Check sheet for the modelled part. Datum: model origin and axes. Units: mm. A direction names the side the tool comes from. Round coordinates to 2 decimals unless told otherwise and drop trailing zeros. Order: outer loops, then holes, each group sorted by start corner. A loop starts at its lowest first (then second) coordinate and runs counter-clockwise, first axis right, second up. Notation, with made-up numbers: (-39, 42.25) -> (-28, 42.25) arc R24 cw to (-28, 61.25) -> close; hole circle Ø7 at (55.5, -33). An arc over 180 degrees is marked (long way). Answer as CSV lines item,"result". Start each with the question number.
from build123d import *

# Parameters (mm, degrees)
ESQUISSE1_R        = 16.5
BOSS_EXTRU_1_DEPTH = 55
CHANFREIN1_SIZE    = 1


with BuildPart() as part:
    # Esquisse1 → Boss.-Extru.1 (new body)
    with BuildSketch(Plane(origin=(0, 0, 0), x_dir=(1, 0, 0), z_dir=(0, 1, 0))):
        with Locations(Location((0, 0, 0), (0, 0, 270))):  # turned: the seam where the file's is
            Circle(ESQUISSE1_R)
    extrude(amount=BOSS_EXTRU_1_DEPTH)

    # Esquisse4 → Révolution1 (revolve)
    with BuildSketch(Plane.XY, mode=Mode.PRIVATE) as r_volution1_sk:
        with BuildLine():
            Line((0, 55), (15, 55))
            ThreePointArc((15, 55), (13.247417463, 61.097125593), (15.610891732, 66.984440383))
            ThreePointArc((15.610891732, 66.984440383), (13.732283635, 73.092812528), (16.248093706, 78.967510676))
            ThreePointArc((16.248093706, 78.967510676), (13.634893892, 84.726953942), (15, 90.902428443))
            Line((15, 90.902428443), (15, 136))
            Line((15, 136), (0, 136))
            Line((0, 136), (0, 55))
        make_face()
    revolve(r_volution1_sk.sketch.rotate(Axis((0, 55, 0), (0, 1, 0)), 90), axis=Axis((0, 55, 0), (0, 1, 0)))  # turned: the seam where the file's is

    # Chanfrein1
    chanfrein1_edges = [part.edges().sort_by_distance(p)[0] for p in [
        (0, 136, 15),
    ]]
    chamfer(chanfrein1_edges, length=CHANFREIN1_SIZE)


solid = part.part
1) Depth check by flat-ended pin: pin 1 Ø4 at (y, z) = (52, 9) entering from -X; pin 2 Ø12 at (x, y) = (-4, 88) entering from -Z; pin 3 Ø8 at (x, y) = (12.5, 68.5) entering from +Z. Enter the tip coordinate at first touch or a pass-through.
2) Section check A-A on z = 0. Record the cut outline in (x, y).
3) Section check B-B on x = 0. Record the cut outline in (y, z), then the cut area to 3 significant figures.
4) Access from +Z, -Z, +X, -X, +Y, -Y to the whole of each face (thin tool, end or side, straight path). Record for faces 4 (the face through (-12.65, 113.26, -8.06)), 5 (the face through (0, 0, 0)).
5) Section check C-C on y = 115. Record the cut outline in (x, z).
6) Section check D-D on y = 32. Record the cut outline in (x, z), then the cut area to 3 significant figures.
7) Mould release check, pull along Y, two halves, no side actions. Record for faces 1 (the face through (-16.108, 27.115, -3.577)), 2 (the face through (-15, 55, 4)), 3 (the face through (0, 136, 0)): released by +Y, released by -Y, zero draft, split by the parting line, or undercut.
8) Material ranges on line 1 along Y through (x, z) = (4, 15); line 2 along Y through (x, z) = (14, 3.5); line 3 along X through (y, z) = (47, 6), recorded low to high.
Solutions:
1,pin 1,"stops at x = -14.94"
1,pin 2,"stops at z = -15"
1,pin 3,"stops at z = 12.9"
2,outline,"(-16.5, 0) -> (16.5, 0) -> (16.5, 55) -> (15, 55) arc R9.77 cw to (15.61, 66.98) arc R9.28 cw to (16.25, 78.97) arc R10 cw to (15, 90.9) -> (15, 135) -> (14, 136) -> (-14, 136) -> (-15, 135) -> (-15, 90.9) arc R10 cw to (-16.25, 78.97) arc R9.28 cw to (-15.61, 66.98) arc R9.77 cw to (-15, 55) -> (-16.5, 55) -> close"
3,outline,"(0, -16.5) -> (55, -16.5) -> (55, -15) arc R9.77 cw to (66.98, -15.61) arc R9.28 cw to (78.97, -16.25) arc R10 cw to (90.9, -15) -> (135, -15) -> (136, -14) -> (136, 14) -> (135, 15) -> (90.9, 15) arc R10 cw to (78.97, 16.25) arc R9.28 cw to (66.98, 15.61) arc R9.77 cw to (55, 15) -> (55, 16.5) -> (0, 16.5) -> close"
3,area,"4,190 mm^2"
4,face 4,"+Y"
4,face 5,"+Z, -Z, +X, -X, -Y"
5,outline,"circle Ø30 at (0, 0)"
6,outline,"circle Ø33 at (0, 0)"
6,area,"855 mm^2"
7,face 1,"zero draft"
7,face 2,"undercut"
7,face 3,"released by +Y"
8,line 1,"y = 0 to 55, 66.88 to 67.1, 78.1 to 79.84"
8,line 2,"y = 0 to 55.92, 65.28 to 69.04, 76.16 to 81.73, 89.8 to 135.57"
8,line 3,"x = -15.37 to 15.37"
